Geometry check sheet. Reference: the model listing, model coordinates, mm. Face numbers are marked on the shaded views. Give positions to 0.01 mm unless a question says otherwise; leave off trailing zeros. Order: outer loops, then holes, each group sorted by start corner. A loop starts at its lowest first (then second) coordinate and runs counter-clockwise, first axis right, second up. Notation, with made-up numbers: M 57,-2.75 L 65,-2.75 A25 ccw 65,18.25 Z; hole C 21.5,61 d6. An arc over 180 degrees is marked long. Put each result on its own line as item: value. Start each with the question number.
Q1. Material ranges on L1, parallel to X at y = 7.2, z = 7.5; L2, parallel to Z at x = 5, y = 6.05; L3, parallel to Z at x = 10, y = 4, recorded low to high.
Q2. Section check A-A on x = 2.75. Record the cut outline in (y, z), then the cut area to 3 significant figures.
Q3. Go/stop test with a flat-tipped pin: pin 1 (3 mm diameter, centred on x = 5, z = 7.5, fed in from -Y). Record where the tip stops, or that it passes through.
Q4. Section check B-B on z = 2.5. Record the cut outline in (x, y), then the cut area to 3 significant figures.
Q5. Mould release check, pull along Z, two halves, no side actions. Record for the marked faces 1, 2 and 3: +Z half, -Z half, draft (parallel to the pull), parting line (faces both ways), or undercut.
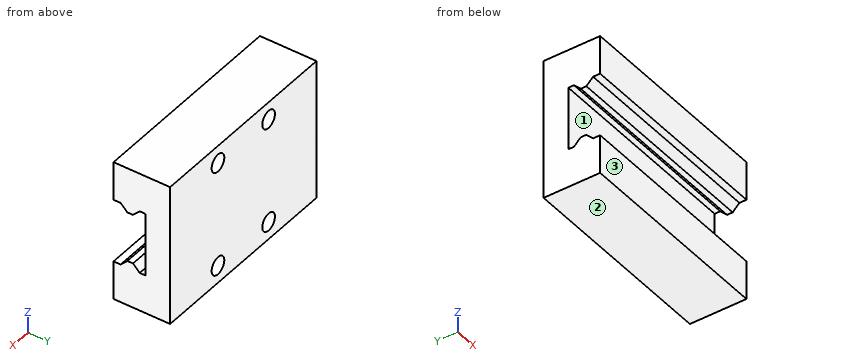
```python
from build123d import *

# Parameters (mm, degrees)
SKETCH_1_W             = 28.9
SKETCH_1_H             = 20
EXTRUDE_1_DEPTH        = 8
CUT_EXTRUDE_1_DEPTH    = 32.610283137
HOLE_WIZARD_M3_1_D     = 2.5
HOLE_WIZARD_M3_1_DEPTH = 3
HOLE_WIZARD_M3_1_TIP   = 0.751075774


with BuildPart() as part:
    # 草图1 → 凸台-拉伸1 (new body)
    with BuildSketch(Plane(origin=(0, 0, 0), x_dir=(1, 0, 0), z_dir=(0, 1, 0))):
        Rectangle(SKETCH_1_W, SKETCH_1_H)
    extrude(amount=EXTRUDE_1_DEPTH)

    # 草图2 → 切除-拉伸1 (cut, through all)
    with BuildSketch(Plane.ZY.offset(14.45)):
        Polygon((-4.5, 0), (-4.5, 1), (-3.55, 1.95), (-3.55, 2.75), (-4.5, 3.7), (-4.5, 4.5), (4.5, 4.5), (4.5, 3.7), (3.55, 2.75), (3.55, 1.95), (4.5, 1), (4.5, 0), align=None)
    extrude(amount=-CUT_EXTRUDE_1_DEPTH, mode=Mode.SUBTRACT)

    # M3 螺纹孔1
    with Locations(Plane(origin=(0, 8, 0), x_dir=(1, 0, 0), z_dir=(0, 1, 0))):
        with Locations((-5, -7.5), (5, -7.5), (5, 7.5), (-5, 7.5)):
            Hole(HOLE_WIZARD_M3_1_D / 2, depth=HOLE_WIZARD_M3_1_DEPTH)
            with Locations((0, 0, -(HOLE_WIZARD_M3_1_DEPTH + HOLE_WIZARD_M3_1_TIP / 2))):  # 118° drill point
                Cone(0, HOLE_WIZARD_M3_1_D / 2, HOLE_WIZARD_M3_1_TIP, mode=Mode.SUBTRACT)


solid = part.part
```
Results found:
1. L1: x = -14.45 to -6.25, -3.75 to 3.75, 6.25 to 14.45
1. L2: z = -10 to -8.75, -6.25 to 6.25, 8.75 to 10
1. L3: z = -10 to -4.5, 4.5 to 10
2. outline: M 0,-10 L 8,-10 L 8,10 L 0,10 L 0,4.5 L 1,4.5 L 1.95,3.55 L 2.75,3.55 L 3.7,4.5 L 4.5,4.5 L 4.5,-4.5 L 3.7,-4.5 L 2.75,-3.55 L 1.95,-3.55 L 1,-4.5 L 0,-4.5 Z
2. area: 123 mm^2
3. pin 1: stops at y = 0
4. outline: M -14.45,4.5 L 14.45,4.5 L 14.45,8 L -14.45,8 Z
4. area: 101 mm^2
5. face 1: undercut
5. face 2: -Z half
5. face 3: draft
